Design review of the part built by this model. Coordinates are the model's own, in mm. Face numbers are marked on the shaded views. A direction names the side the tool comes from. Round coordinates to 2 decimals unless told otherwise and drop trailing zeros. Write each loop counter-clockwise with the first axis right and the second up, starting at its lowest first coordinate (ties: lowest second). Pieces come first, ordered by that corner, then holes. Notation, with made-up numbers: (-38.75, 58.5) -> (8.25, 58.5) arc R23 ccw to (8.25, 91.5) -> close; hole circle Ø6 at (7, -8). An arc over 180 degrees is marked (long way). Write item = value, one per line. Start each with the question number.
Item 1: For pin 1 Ø4.5 at (x, y) = (0, 0) entering from -Z; pin 2 Ø0.8 at (y, z) = (22.5, 1) entering from +X; pin 3 Ø0.8 at (y, z) = (21, 0.5) entering from -X; pin 4 Ø1 at (y, z) = (-5, 0.5) entering from +X, all flat-tipped, find the tip position at first contact; note any pin that passes through.
Item 2: Mouldability with a two-part tool opening along Y and no side actions: class the marked faces 3, 4 and 5 as released by +Y, released by -Y, zero draft, split by the parting line, or undercut.
Item 3: Machinability: for the marked faces 1 and 2, which of the approach directions +Z, -Z, +X, -X, +Y, -Y give a long, thin tool a straight path to every point of the face, cutting with its end or side? Answer none if there is none.
Item 4: Add section A-A, the plane y = 19. State the section outline as (x, z) points.
Item 5: To check wall thickness, follow L1, parallel to X at y = 7, z = 0.55; L2, parallel to X at y = 1.5, z = 0.5; L3, parallel to X at y = 26.5, z = 2.2. State the ranges of each line that lie inside material, in increasing order.
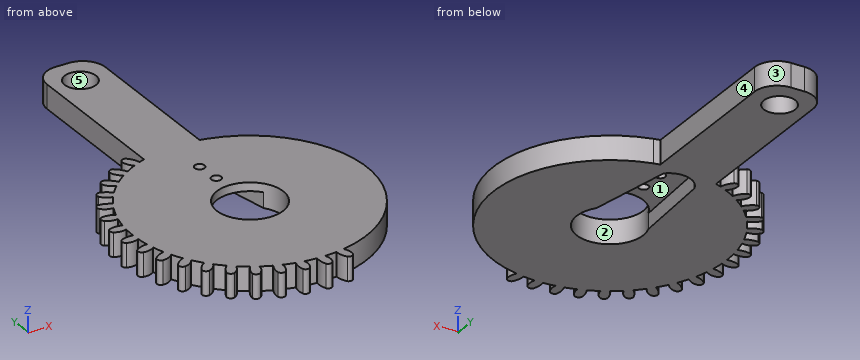
from build123d import *

# Parameters (mm, degrees)
SKETCH1_R           = 13
BOSS_EXTRUDE1_DEPTH = 2.65
BOSS_EXTRUDE2_DEPTH = 2.65
CIRPATTERN1_COUNT   = 37
CUT_EXTRUDE1_DEPTH  = 6
SKETCH5_W           = 6.5
SKETCH5_H           = 20
BOSS_EXTRUDE3_DEPTH = 2.65
FILLET1_R           = 2.5
SKETCH6_R           = 3.7
CUT_EXTRUDE2_DEPTH  = 36.535053909
SKETCH8_R           = 1.75
CUT_EXTRUDE4_DEPTH  = 36.535053909
CUT_EXTRUDE5_DEPTH  = 1.7
SKETCH9_R           = 0.55
CUT_EXTRUDE6_DEPTH  = 36.476859448


with BuildPart() as part:
    # Sketch1 → Boss-Extrude1 (new body)
    with BuildSketch(Plane.XY):
        Circle(SKETCH1_R)
    extrude(amount=BOSS_EXTRUDE1_DEPTH)

    # Sketch2 → Boss-Extrude2 (add)
    with BuildSketch(Plane.XY.offset(2.65)):
        with BuildLine():
            Line((-1.407237761, 12.923609476), (-0.564746485, 12.987727338))
            ThreePointArc((-0.564746485, 12.987727338), (-0.590917928, 13.726605325), (-0.839716114, 14.422827334))
            ThreePointArc((-0.839716114, 14.422827334), (-1.250735375, 14.570045044), (-1.59276063, 14.298699117))
            ThreePointArc((-1.59276063, 14.298699117), (-1.655805876, 13.590133338), (-1.407237761, 12.923609476))
        make_face()
    boss_extrude2 = extrude(amount=-BOSS_EXTRUDE2_DEPTH)

    # CirPattern1: Boss-Extrude2 ×37 about axis
    cirpattern1_axis = Axis((-0.00317711, 0.03890501, 0), (0, 0, 1))
    for i in range(1, CIRPATTERN1_COUNT):
        add(boss_extrude2.rotate(cirpattern1_axis, i * 360 / CIRPATTERN1_COUNT))

    # Sketch3 → Cut-Extrude1 (cut)
    with BuildSketch(Plane.XY.offset(2.65)):
        with BuildLine():
            ThreePointArc((2.539809494, -12.749484999), (12.964979242, -0.216908767), (2.964875647, 12.657389636))
            ThreePointArc((2.964875647, 12.657389636), (2.750073389, 13.993219942), (3.542759924, 15.089682744))
            ThreePointArc((3.542759924, 15.089682744), (15.464629435, -0.258728814), (3.036006853, -15.199747879))
            ThreePointArc((3.036006853, -15.199747879), (3.295374232, -13.871850601), (2.539809494, -12.749484999))
        make_face()
    extrude(amount=-CUT_EXTRUDE1_DEPTH, mode=Mode.SUBTRACT)

    # Sketch5 → Boss-Extrude3 (add)
    with BuildSketch(Plane.XY.offset(2.65)):
        with Locations((-0.96169727, 22.298845722)):
            Rectangle(SKETCH5_W, SKETCH5_H)
    extrude(amount=-BOSS_EXTRUDE3_DEPTH)

    # Fillet1
    fillet1_edges = [part.edges().sort_by_distance(p)[0] for p in [
        (2.28830273, 32.298845722, 1.325),
        (-4.21169727, 32.298845722, 1.325),
    ]]
    fillet(fillet1_edges, radius=FILLET1_R)

    # Sketch6 → Cut-Extrude2 (cut, through all)
    with BuildSketch(Plane(origin=(0, 0, 0), x_dir=(-1, 0, 0), z_dir=(0, 0, -1))):
        Circle(SKETCH6_R)
    extrude(amount=-CUT_EXTRUDE2_DEPTH, mode=Mode.SUBTRACT)

    # Sketch8 → Cut-Extrude4 (cut, through all)
    with BuildSketch(Plane(origin=(0, 0, 0), x_dir=(-1, 0, 0), z_dir=(0, 0, -1))):
        with Locations((1.101176672, 28.798845722)):
            Circle(SKETCH8_R)
    extrude(amount=-CUT_EXTRUDE4_DEPTH, mode=Mode.SUBTRACT)

    # Sketch7 → Cut-Extrude5 (cut)
    with BuildSketch(Plane(origin=(0, 0, 0), x_dir=(-1, 0, 0), z_dir=(0, 0, -1))):
        with BuildLine():
            Line((3.457410227, 1.317692879), (2.9338417, 10.436920645))
            ThreePointArc((2.9338417, 10.436920645), (1.193583976, 12.06013788), (-1.112499205, 11.472505769))
            Line((-1.112499205, 11.472505769), (-2.915695151, 2.277876596))
            ThreePointArc((-2.915695151, 2.277876596), (0.551227719, 3.658708516), (3.457410227, 1.317692879))
        make_face()
    extrude(amount=-CUT_EXTRUDE5_DEPTH, mode=Mode.SUBTRACT)

    # Sketch9 → Cut-Extrude6 (cut, through all)
    with BuildSketch(Plane(origin=(0, 0, 1.7), x_dir=(-1, 0, 0), z_dir=(0, 0, -1))):
        with Locations((0.330807323, 5.53577119)):
            Circle(SKETCH9_R)
        with Locations((0.490803437, 8.294426445)):
            Circle(SKETCH9_R)
    extrude(amount=-CUT_EXTRUDE6_DEPTH, mode=Mode.SUBTRACT)


solid = part.part
Result set:
q1.pin_1 = through
q1.pin_2 = 2.29
q1.pin_3 = -4.21
q1.pin_4 = 12.16
q2.face_3 = released by +Y
q2.face_4 = zero draft
q2.face_5 = undercut
q3.face_1 = -Z
q3.face_2 = +Z, -Z
q4.outline = (-4.21, 0) -> (2.29, 0) -> (2.29, 2.65) -> (-4.21, 2.65) -> close
q5.L1 = -10.95 to -3.13, 1.99 to 10.92
q5.L2 = -14.29 to -3.45, 3.38 to 12.88
q5.L3 = -4.21 to 2.29
